from build123d import *

# Parameters (mm, degrees)
BOX_W           = 22
BOX_H           = 40
BOX_DEPTH       = 22
SKETCH_W        = 18
SKETCH_H        = 18
POCKET_DEPTH    = 40.001
SKETCH001_W     = 10
SKETCH001_H     = 10
POCKET001_DEPTH = 4.001
SKETCH002_R     = 1.5
POCKET002_DEPTH = 22.001


with BuildPart() as part:
    # Box → Box (new body)
    with BuildSketch(Plane.XY):
        with Locations((11, 20)):
            Rectangle(BOX_W, BOX_H)
    extrude(amount=BOX_DEPTH)

    # Sketch → Pocket (cut, through all)
    with BuildSketch(Plane.XZ):
        with Locations((9, 9)):
            Rectangle(SKETCH_W, SKETCH_H)
    extrude(amount=-POCKET_DEPTH, mode=Mode.SUBTRACT)

    # Sketch001 → Pocket001 (cut, through all)
    with BuildSketch(Plane(origin=(18, 0, 0), x_dir=(0, -1, 0), z_dir=(-1, 0, 0))):
        with Locations((-20, 9.5)):
            Rectangle(SKETCH001_W, SKETCH001_H)
    extrude(amount=-POCKET001_DEPTH, mode=Mode.SUBTRACT)

    # Sketch002 → Pocket002 (cut, through all)
    with BuildSketch(Plane.YZ.offset(22)):
        with Locations((4, 9.5)):
            Circle(SKETCH002_R)
        with Locations((11, 9.5)):
            Circle(SKETCH002_R)
        with Locations((29, 9.5)):
            Circle(SKETCH002_R)
        with Locations((36, 9.5)):
            Circle(SKETCH002_R)
    extrude(amount=-POCKET002_DEPTH, mode=Mode.SUBTRACT)


solid = part.part
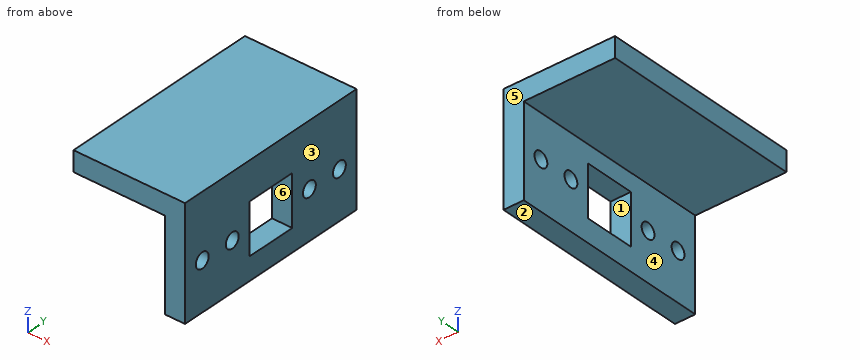
Here's how the part is built. I have some questions about the finished solid (model axes, mm). Face numbers are marked on the shaded views. A direction names the side the tool comes from. Give positions to 0.01 mm unless a question says otherwise; leave off trailing zeros. Loops run counter-clockwise (first coordinate to the right, second up) from the corner with the lowest first, then second, coordinate; pieces in that order, holes last. Notation, with made-up numbers: (15, 12.25) -> (52, 12.25) arc R12 cw to (52, 24.25) -> close; hole circle Ø10 at (24.25, -30). An arc over 180 degrees is marked (long way). One line per item, written item: value.
Q1. I'm going to push flat-ended pins straight in: pin 1 Ø5 at (y, z) = (4, 9.5) entering from -X; pin 2 Ø8 at (x, y) = (4.5, 35.5) entering from -Z. Where does each tip first touch, or does it pass through?
Answers follow:
pin 1: x = 18
pin 2: z = 18
Q2. Suppose I cut it at A-A on y = 4. Please give me the cut outline in (x, z).
Answers follow:
outline: (0, 18) -> (18, 18) -> (18, 11) -> (22, 11) -> (22, 22) -> (0, 22) -> close; (18, 0) -> (22, 0) -> (22, 8) -> (18, 8) -> close
Q3. We'd pull the mould along Z, two halves only. Please class the marked faces 1, 2 and 3: pulls with the +Z half, pulls with the -Z half, needs draft (parallel to the pull), parting line crosses it, or undercut.
Answers follow:
face 1: undercut
face 2: pulls with the -Z half
face 3: needs draft
Q4. If I drill on line 1 along Z through (x, y) = (20.5, 4); line 2 along Z through (x, y) = (20, 18.5); line 3 along X through (y, z) = (28, 14), over which ranges is the centre line in solid material (lowest first)?
Answers follow:
line 1: 0 to 8, 11 to 22
line 2: 0 to 4.5, 14.5 to 22
line 3: 18 to 22
Q5. On a 3-axis mill with a long thin cutter (end or side, diameter ignored), from which of +Z, -Z, +X, -X, +Y, -Y can I reach the whole of each face in a straight line? I mean the marked faces 4, 5 and 6. Say none if no direction works.
Answers follow:
face 4: -Z, -X, +Y, -Y
face 5: +Z, -Z, +X, -X, +Y
face 6: +X, -X
Q6. Suppose I cut it at D-D on z = 10. Please give me the cut outline in (x, y).
Answers follow:
outline: (18, 0) -> (22, 0) -> (22, 2.59) -> (18, 2.59) -> close; (18, 5.41) -> (22, 5.41) -> (22, 9.59) -> (18, 9.59) -> close; (18, 12.41) -> (22, 12.41) -> (22, 15) -> (18, 15) -> close; (18, 25) -> (22, 25) -> (22, 27.59) -> (18, 27.59) -> close; (18, 30.41) -> (22, 30.41) -> (22, 34.59) -> (18, 34.59) -> close; (18, 37.41) -> (22, 37.41) -> (22, 40) -> (18, 40) -> close
Q7. Suppose I cut it at B-B on z = 7.5. Please give me the cut outline in (x, y), then the cut area to 3 significant figures.
Answers follow:
outline: (18, 0) -> (22, 0) -> (22, 15) -> (18, 15) -> close; (18, 25) -> (22, 25) -> (22, 40) -> (18, 40) -> close
area: 120 mm^2
Q8. Suppose I cut it at C-C on x = 20.75. Please give me the cut outline in (y, z).
Answers follow:
outline: (0, 0) -> (40, 0) -> (40, 22) -> (0, 22) -> close; hole circle Ø3 at (4, 9.5); hole circle Ø3 at (11, 9.5); hole (15, 4.5) -> (25, 4.5) -> (25, 14.5) -> (15, 14.5) -> close; hole circle Ø3 at (29, 9.5); hole circle Ø3 at (36, 9.5)
